Read the model definition and answer for the solid it produces. Units are mm, in the model's axes. Face numbers are marked on the shaded views. A direction names the side the tool comes from. Round coordinates to 2 decimals unless told otherwise and drop trailing zeros. Order: outer loops, then holes, each group sorted by start corner. A loop starts at its lowest first (then second) coordinate and runs counter-clockwise, first axis right, second up. Notation, with made-up numbers: (76.25, 8) - (89.25, 8) arc R14 cw to (89.25, 25) - close; hole circle Ø9 at (70, 80.25). An arc over 180 degrees is marked (long way). Answer as a JSON object with one key per item and string values. Group by question number.
Q1. A cutting plane is placed at A-A on x = -208. Determine the outline of the cut face in (y, z).
Q2. A cutting plane is placed at B-B on x = -550.5. Determine the outline of the cut face in (y, z), and give its area (3 significant figures).
Q3. A tool of negligible diameter and unlimited length cuts with its end or side. For the marked faces 1 and 2, from which of +Z, -Z, +X, -X, +Y, -Y can it reach the whole face along a straight path? Write none if from no direction.
Q4. A cutting plane is placed at C-C on x = -744. Determine the outline of the cut face in (y, z), and give its area (3 significant figures).
Q5. Given pin 1 Ø3 at (x, y) = (-515, -6) entering from -Z; pin 2 Ø17 at (x, z) = (-826.5, 25) entering from +Y; pin 3 Ø15 at (x, z) = (-491.5, 35) entering from -Y, each flat-ended and moving along its own axis, determine where each tip first touches the part or whether it passes through.
Q6. Consider line 1 (Z direction, x = -826.5, y = -7.85); line 2 (Y direction, x = -379.5, z = 20); line 3 (Y direction, x = -757, z = 17). Determine where each line is inside the solid, lowest interval first.
```python
from build123d import *

# Parameters (mm, degrees)
SM_BASE_FLANGE_1_DEPTH = 50
SKETCH_4_R             = 6.9
CUT_EXTRUDE_3_DEPTH    = 10
SKETCH_5_R             = 6.5
CUT_EXTRUDE_4_DEPTH    = 10
OTHER_START            = -10
OTHER_1_DEPTH          = 10
CUT_EXTRUDE_5_DEPTH    = 10


# Read off the part's stored shape, not the designer's step: Затупленный угол1
# Sheet-metal steps are written as plain solids
with BuildPart() as part:
    # Sketch 1 → Базовая кромка1 (new body)
    with BuildSketch(Plane.XY):
        with BuildLine():
            Line((-851.5, -5), (-791.936609429, -5))
            ThreePointArc((-791.936609429, -5), (-791.500415555, -4.990482216), (-791.065052002, -4.961946981))
            Line((-791.065052002, -4.961946981), (-735.002160484, -0.057079529))
            ThreePointArc((-735.002160484, -0.057079529), (-734.349115153, -0.014276676), (-733.694824343, 0))
            Line((-733.694824343, 0), (0, 0))
            Line((0, 0), (0, -5))
            Line((0, -5), (-733.694824343, -5))
            ThreePointArc((-733.694824343, -5), (-734.131018216, -5.009517784), (-734.56638177, -5.038053019))
            Line((-734.56638177, -5.038053019), (-790.629273288, -9.942920471))
            ThreePointArc((-790.629273288, -9.942920471), (-791.282318619, -9.985723324), (-791.936609429, -10))
            Line((-791.936609429, -10), (-851.5, -10))
            Line((-851.5, -10), (-851.5, -5))
        make_face()
    extrude(amount=SM_BASE_FLANGE_1_DEPTH)

    # Эскиз4 → Вырез-Вытянуть3 (cut)
    with BuildSketch(Plane(origin=(0, 0, 0), x_dir=(1, 0, 0), z_dir=(0, 1, 0))):
        with Locations(Location((-208, -25, 0), (0, 0, 270))):
            Circle(SKETCH_4_R)
        with BuildLine():
            Line((-309.5, -31.5), (-316.5, -31.5))
            ThreePointArc((-316.5, -31.5), (-323, -25), (-316.5, -18.5))
            Line((-316.5, -18.5), (-309.5, -18.5))
            ThreePointArc((-309.5, -18.5), (-303, -25), (-309.5, -31.5))
        make_face()
    extrude(amount=-CUT_EXTRUDE_3_DEPTH, mode=Mode.SUBTRACT)

    # Эскиз5 → Вырез-Вытянуть4 (cut)
    with BuildSketch(Plane(origin=(0, -5, 0), x_dir=(1, 0, 0), z_dir=(0, 1, 0))):
        with Locations(Location((-826.5, -25, 0), (0, 0, 180))):
            Circle(SKETCH_5_R)
    extrude(amount=-CUT_EXTRUDE_4_DEPTH, mode=Mode.SUBTRACT)

    # Other 1 outline → Other 1 (cut)
    with BuildSketch(Plane(origin=(0, 0, 0), x_dir=(1, 0, 0), z_dir=(0, 1, 0)).offset(OTHER_START)):
        Polygon((0, 0), (-5, 0), (0, -5), align=None)
        Polygon((0, -50), (0, -45), (-5, -50), align=None)
        Polygon((-851.5, 0), (-851.5, -5), (-846.5, 0), align=None)
        Polygon((-846.5, -50), (-851.5, -45), (-851.5, -50), align=None)
    extrude(amount=OTHER_1_DEPTH, mode=Mode.SUBTRACT)

    # Эскиз6 → Вырез-Вытянуть5 (cut)
    with BuildSketch(Plane(origin=(0, 0, 0), x_dir=(1, 0, 0), z_dir=(0, 1, 0))):
        with BuildLine():
            Line((-19, -31), (-31, -31))
            ThreePointArc((-31, -31), (-37, -25), (-31, -19))
            Line((-31, -19), (-19, -19))
            ThreePointArc((-19, -19), (-13, -25), (-19, -31))
        make_face()
    extrude(amount=-CUT_EXTRUDE_5_DEPTH, mode=Mode.SUBTRACT)


solid = part.part
```
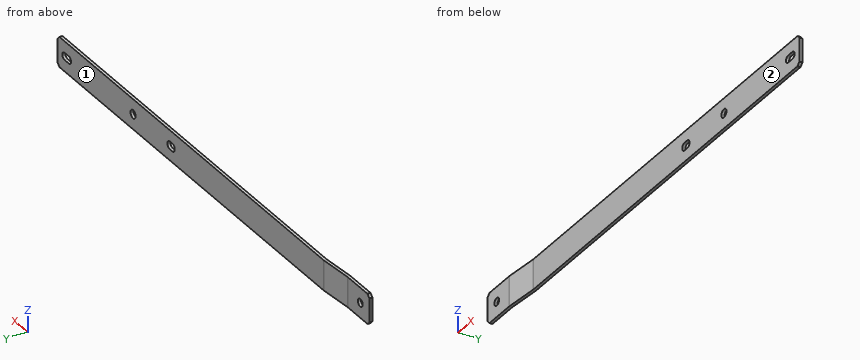
Result set:
{
 "1": {"outline": "(-5, 0) - (0, 0) - (0, 18.1) - (-5, 18.1) - close; (-5, 31.9) - (0, 31.9) - (0, 50) - (-5, 50) - close"},
 "2": {"outline": "(-5, 0) - (0, 0) - (0, 50) - (-5, 50) - close", "area": "250 mm²"},
 "3": {"face 1": "+Z, -Z, +X, -X, +Y", "face 2": "+Z, -Z, +X, -Y"},
 "4": {"outline": "(-5.86, 0) - (-0.84, 0) - (-0.84, 50) - (-5.86, 50) - close", "area": "251 mm²"},
 "5": {"pin 1": "stops at z = 0", "pin 2": "stops at y = -5", "pin 3": "stops at y = -5"},
 "6": {"line 1": "z = 0 to 18.5, 31.5 to 50", "line 2": "y = -5 to 0", "line 3": "y = -7 to -1.98"}
}
